Could you check a few things on this drawing? It's one solid part, dimensions in mm from its lowest x, y, z. Round coordinates to 2 decimals unless told otherwise and drop trailing zeros. Loops run counter-clockwise (first coordinate to the right, second up) from the corner with the lowest first, then second, coordinate; pieces in that order, holes last. Notation, with made-up numbers: (79.25, 17.25) -> (91.25, 17.25) arc R25 cw to (91.25, 53.25) -> close; hole circle Ø11 at (81.25, -13.5). An arc over 180 degrees is marked (long way). Write each question's results on one line, items separated by ' | '.
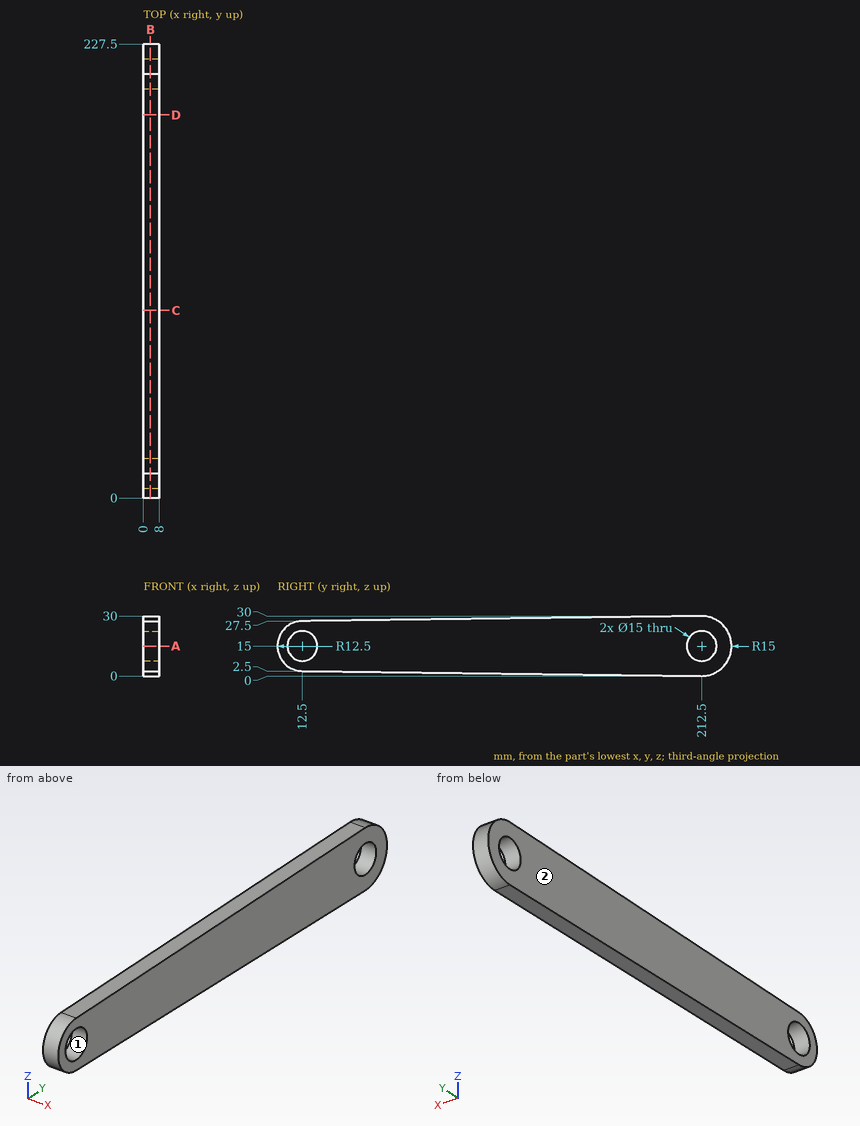
1) I want a section at D-D, the plane y = 192. Write out the boundary of the cut face in (x, z), plus the area to 3 significant figures.
Model answer:
outline: (0, 0.26) -> (8, 0.26) -> (8, 29.74) -> (0, 29.74) -> close | area: 236 mm2
2) I need wall thicknesses on line 1 (Y direction, x = 6.25, z = 15); line 2 (Y direction, x = 3, z = 16); line 3 (Y direction, x = 7.5, z = 23.5). Which ranges of each line are inside material? Lowest first, please.
Model answer:
line 1: y = 0 to 5, 20 to 205, 220 to 227.5 | line 2: y = 0.04 to 5.07, 19.93 to 205.07, 219.93 to 227.47 | line 3: y = 3.33 to 224.86
3) I'm going to push flat-ended pins straight in: pin 1 (4 mm diameter, centred on x = 6.5, z = 9, fed in from +Y); pin 2 (3 mm diameter, centred on x = 5, z = 17.5, fed in from -Y); pin 3 (1.5 mm diameter, centred on x = 1, y = 107.5, fed in from -Z). Where does each tip first touch, or does it pass through?
Model answer:
pin 1: stops at y = 226.96 | pin 2: stops at y = 0.04 | pin 3: stops at z = 1.3
4) I want a section at B-B, the plane x = 3.5. Write out the boundary of the cut face in (y, z), plus the area to 3 significant figures.
Model answer:
outline: (12.5, 2.5) -> (212.5, 0) arc R15 ccw to (212.5, 30) -> (12.5, 27.5) arc R12.5 ccw to start; hole circle Ø15 at (12.5, 15); hole circle Ø15 at (212.5, 15) | area: 5,750 mm2
5) I want a section at A-A, the plane z = 15. Write out the boundary of the cut face in (x, y).
Model answer:
outline: (0, 0) -> (8, 0) -> (8, 5) -> (0, 5) -> close; (0, 20) -> (8, 20) -> (8, 205) -> (0, 205) -> close; (0, 220) -> (8, 220) -> (8, 227.5) -> (0, 227.5) -> close
6) I want a section at C-C, the plane y = 94. Write out the boundary of the cut face in (x, z).
Model answer:
outline: (0, 1.48) -> (8, 1.48) -> (8, 28.52) -> (0, 28.52) -> close
7) If we mould it in two halves opening along Z, with no side actions, what happens to the marked faces 1 and 2? For each: released by +Z, released by -Z, zero draft, split by the parting line, or undercut.
Model answer:
face 1: undercut | face 2: zero draft
